Could you check a few things on this model? Use its own coordinates, in mm. A direction names the side the tool comes from. Give positions to 0.01 mm unless a question says otherwise; leave off trailing zeros. Loops run counter-clockwise (first coordinate to the right, second up) from the corner with the lowest first, then second, coordinate; pieces in that order, holes last. Notation, with made-up numbers: M 43.5,-36.5 L 94.5,-36.5 A16 ccw 94.5,-17.5 Z; hole C -12.5,50.25 d8. An arc over 180 degrees is marked long. Return JSON: item names as keys, results as strings. Group by question number.
1. If we section it at C-C (x = 137.5): Write out the boundary of the cut face in (y, z), plus the area to 3 significant figures.
2. If we section it at B-B (y = 18): Write out the boundary of the cut face in (x, z), plus the area to 3 significant figures.
3. If we mould it in two halves opening along X, with no side actions, what happens to faces 5 (the flat face through (163, 2, -91)), 6 (the flat face through (14.35, 2, -50)), 7 (the flat face through (98, 13, 0))? For each: +X half, -X half, draft (parallel to the pull), parting line (faces both ways), or undercut.
4. For pin 1 (8 mm diameter, centred on x = 70, z = -27.5, fed in from +Y); pin 2 (1.5 mm diameter, centred on y = 1, z = -47, fed in from +X), each with a flat end and sliding along its axis, tell me the tip position at first contact or that it passes through.
5. Please list where these lines run through material, in increasing order: line 1 (Z direction, x = 115, y = 2.3); line 2 (Z direction, x = 146.5, y = 6.5); line 3 (Y direction, x = 85.5, z = -19.5).
6. For faces 1 (the cylindrical face through (155.25, 17.88, -1.48)), 2 (the flat face through (151, 33, -99)), 3 (the flat face through (147, 1, -67.5)), 4 (the flat face through (98, 15, -97)), which set-ups out of +Z, -Z, +X, -X, +Y, -Y let a thin tool reach every point of the face, with its end or its side?
7. If we section it at D-D (x = 23): Write out the boundary of the cut face in (y, z).
8. If we section it at A-A (y = 7.5): Write out the boundary of the cut face in (x, z), plus the area to 3 significant figures.
Autodesk Inventor part; units mm, degrees
ref_plane "YZ Plane" through (0, 0, 0) normal (1, 0, 0) x (0, 1, 0)
ref_plane "XZ Plane" through (0, 0, 0) normal (0, 1, 0) x (-1, 0, 0)
ref_plane "XY Plane" through (0, 0, 0) normal (0, 0, 1) x (1, 0, 0)
sketch "Náčrt1" plane through (0, 0, 0) normal (1, 0, 0) x (0, 1, 0)
  line L0 (0, 0) -> (0, -100)
  line L1 (0, -100) -> (33, -100)
  line L2 (33, -100) -> (33, -97)
  line L3 (33, -97) -> (3, -97)
  line L4 (3, -97) -> (3, -3)
  line L5 (3, -3) -> (33, -3)
  line L6 (33, -3) -> (33, 0)
  line L7 (33, 0) -> (0, 0)
  dimension "d0" = 100
  dimension "d1" = 33
  dimension "d2" = 3
  dimension "d3" = 30
  dimension "d4" = 94
  dimension "d5" = 30
  dimension "d6" = 3
extrude "Vysunutí1" add sketch "Náčrt1" along normal blind 160
sketch "Náčrt4" plane through (0, 3, -3) normal (0, 1, 0) x (1, 0, 0)
  line L0 (0, 94) -> (0, 0)
  line L1 (0, 0) -> (160, 0)
  line L2 (160, 94) -> (160, 0)
  line L3 (0, 94) -> (160, 94)
  line L4 (14.35, 52.65) -> (25.65, 52.65)
  line L5 (25.65, 52.65) -> (25.65, 41.35)
  line L6 (25.65, 41.35) -> (14.35, 41.35)
  line L7 (14.35, 41.35) -> (14.35, 52.65)
  line L8 (0, 97) -> (160, 97)
  point P0 (0, -3)
  point P1 (20, 41.35)
  point P2 (14.35, 47)
  dimension "d104" = 11.3
  dimension "d105" = 11.3
  dimension "d106" = 50
  dimension "d107" = 140
extrude "Vysunutí4" cut sketch "Náčrt4" against normal through all contours L4 L5 L6 L7
sketch "Náčrt7" plane through (0, 0, -100) normal (0, -1, 0) x (1, 0, 0)
  line L0 (0, 100) -> (0, 0)
  line L1 (0, 0) -> (160, 0)
  line L2 (160, 100) -> (160, 0)
  line L3 (0, 100) -> (160, 100)
  circle A0 centre (115, 90) radius 2.25
  circle A1 centre (115, 10) radius 2.25
  dimension "d76" = 4.5
  dimension "d77" = 4.5
  dimension "d78" = 10
  dimension "d79" = 10
  dimension "d80" = 115
  dimension "d81" = 115
extrude "Vysunutí7" cut sketch "Náčrt7" against normal through all contours A0 | A1
sketch "Náčrt8" plane through (0, 0, -100) normal (0, 0, -1) x (-1, 0, 0)
  line L0 (0, 0) -> (0, 33)
  line L1 (0, 33) -> (-160, 33)
  line L2 (-160, 0) -> (-160, 33)
  line L3 (0, 0) -> (-160, 0)
  line L4 (0, 3) -> (-160, 3)
  line L5 (0, 0) -> (0, 33)
  line L6 (0, 3) -> (-140, 33)
  line L7 (0, 33) -> (-160, 33)
  line L8 (0, 3) -> (0, 33)
  line L9 (0, 33) -> (-140, 33)
  dimension "d85" = 140
  dimension "d86" = 30
extrude "Vysunutí8" cut sketch "Náčrt8" against normal through all contours L6 L1 L0
sketch "Náčrt9" plane through (0, 0, -100) normal (0, -1, 0) x (1, 0, 0)
  circle A0 centre (115, 90) radius 2.25
  circle A1 centre (115, 10) radius 2.25
  line L0 (0, 100) -> (0, 0)
  line L1 (0, 0) -> (160, 0)
  line L2 (160, 100) -> (160, 0)
  line L3 (0, 100) -> (160, 100)
  line L4 (130, 67.5) -> (160, 67.5)
  line L5 (160, 67.5) -> (160, 32.5)
  line L6 (160, 32.5) -> (130, 32.5)
  line L7 (130, 32.5) -> (130, 67.5)
  line L8 (160, 100) -> (160, 0)
  point P0 (130, 50)
  dimension "d90" = 35
  dimension "d91" = 50
  dimension "d92" = 30
  dimension "d93" = 30
extrude "Vysunutí9" cut sketch "Náčrt9" against normal through all contours L2 L6 L7 L4
sketch "Náčrt10" plane through (160, 0, 0) normal (1, 0, 0) x (0, 0, -1)
  line L0 (67.5, 3) -> (67.5, 0)
  line L1 (67.5, 0) -> (100, 0)
  line L2 (100, 0) -> (100, 33)
  line L3 (100, 33) -> (97, 33)
  line L4 (97, 33) -> (97, 3)
  line L5 (97, 3) -> (67.5, 3)
  line L6 (32.5, 0) -> (32.5, 3)
  line L7 (32.5, 3) -> (3, 3)
  line L8 (3, 3) -> (3, 33)
  line L9 (3, 33) -> (0, 33)
  line L10 (0, 33) -> (0, 0)
  line L11 (0, 0) -> (32.5, 0)
extrude "Vysunutí10" add sketch "Náčrt10" along normal blind 3
sketch "Náčrt11" plane through (0, 0, 0) normal (0, 0, 1) x (1, 0, 0)
  line L0 (140, 33) -> (0, 3)
  line L1 (0, 3) -> (0, 0)
  line L2 (0, 0) -> (163, 0)
  line L3 (163, 33) -> (163, 0)
  line L4 (140, 33) -> (163, 33)
  arc A0 (150, 12.75) -> (150, 23.25) centre (150, 18) ccw
  arc A1 (140, 23.25) -> (140, 12.75) centre (140, 18) ccw
  line L5 (150, 12.75) -> (140, 12.75)
  line L6 (140, 23.25) -> (150, 23.25)
  dimension "d98" = 10.5
  dimension "d99" = 10.5
  dimension "d100" = 10
  dimension "d101" = 13
  dimension "d108" = 15
extrude "Vysunutí11" cut sketch "Náčrt11" against normal through all contours L5 A1 L6 A0
properties part number "U-profil 100x40 - pod case"
Answer:
{
 "1": {"outline": "M 0,-100 L 13.38,-100 L 13.38,-97 L 3,-97 L 3,-67.5 L 0,-67.5 Z; M 0,-32.5 L 3,-32.5 L 3,-3 L 13.38,-3 L 13.38,0 L 0,0 Z; M 22.62,-100 L 32.46,-100 L 32.46,-97 L 22.62,-97 Z; M 22.62,-3 L 32.46,-3 L 32.46,0 L 22.62,0 Z", "area": "316 mm²"},
 "2": {"outline": "M 70,-100 L 134.75,-100 L 134.75,-97 L 70,-97 Z; M 70,-3 L 134.75,-3 L 134.75,0 L 70,0 Z; M 155.25,-100 L 163,-100 L 163,-97 L 155.25,-97 Z; M 155.25,-3 L 163,-3 L 163,0 L 155.25,0 Z", "area": "435 mm²"},
 "3": {"face 5": "+X half", "face 6": "undercut", "face 7": "draft"},
 "4": {"pin 1": "stops at y = 3", "pin 2": "stops at x = 130"},
 "5": {"line 1": "z = -100 to -92.25, -87.75 to -12.25, -7.75 to 0", "line 2": "z = -100 to -97, -3 to 0", "line 3": "y = 0 to 3"},
 "6": {"face 1": "+Z, -Z", "face 2": "+Z, -Z, +X, -X, +Y", "face 3": "+X, +Y, -Y", "face 4": "+X, -X, +Y"},
 "7": {"outline": "M 0,-100 L 7.93,-100 L 7.93,-97 L 3,-97 L 3,-55.65 L 0,-55.65 Z; M 0,-44.35 L 3,-44.35 L 3,-3 L 7.93,-3 L 7.93,0 L 0,0 Z"},
 "8": {"outline": "M 21,-100 L 163,-100 L 163,-97 L 21,-97 Z; M 21,-3 L 163,-3 L 163,0 L 21,0 Z", "area": "852 mm²"}
}
